from build123d import *

# Parameters (mm, degrees)
SKETCH_1_R              = 25
SKETCH_1_R_2            = 20
EXTRUDE_1_DEPTH         = 1
HOLE_WIZARD_3_9_3_9_1_D = 3.9
SKETCH_4_R              = 2
CUT_EXTRUDE_1_DEPTH     = 10


with BuildPart() as part:
    # 草图1 → 凸台-拉伸1 (new body)
    with BuildSketch(Plane.XY):
        with BuildLine():
            Line((-62.449979984, 62), (62.449979984, 62))
            ThreePointArc((62.449979984, 62), (0, -88), (-62.449979984, 62))
        make_face()
        Circle(SKETCH_1_R, mode=Mode.SUBTRACT)
        with Locations((54.772, 35)):
            Circle(SKETCH_1_R_2, mode=Mode.SUBTRACT)
        with Locations(Location((-54.772, 35, 0), (0, 0, 180))):
            Circle(SKETCH_1_R_2, mode=Mode.SUBTRACT)
        with Locations((35, -54.772255751)):
            Circle(SKETCH_1_R_2, mode=Mode.SUBTRACT)
        with Locations((-35, -54.772255751)):
            Circle(SKETCH_1_R_2, mode=Mode.SUBTRACT)
    extrude(amount=EXTRUDE_1_DEPTH)

    # Ø3.9 (3.9) 直径孔1 (through all)
    with Locations(Plane(origin=(0, 0, 0), x_dir=(-1, 0, 0), z_dir=(0, 0, -1))):
        with Locations((-77, 26), (-77, -27), (77, -27), (77, 26)):
            Hole(HOLE_WIZARD_3_9_3_9_1_D / 2)

    # 草图4 → 切除-拉伸1 (cut)
    with BuildSketch(Plane.XY.offset(1)):
        with Locations((-60, 0)):
            Circle(SKETCH_4_R)
        with Locations((0, 40)):
            Circle(SKETCH_4_R)
        with Locations((60, 0)):
            Circle(SKETCH_4_R)
        with Locations((0, -60)):
            Circle(SKETCH_4_R)
    extrude(amount=-CUT_EXTRUDE_1_DEPTH, mode=Mode.SUBTRACT)


solid = part.part
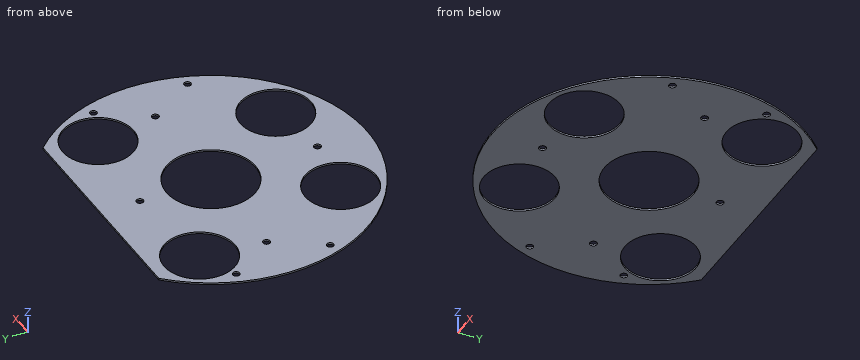
CAD build for the part. Positions are in the model's coordinates, mm. Round coordinates to 2 decimals unless told otherwise and drop trailing zeros. Order: outer loops, then holes, each group sorted by start corner. A loop starts at its lowest first (then second) coordinate and runs counter-clockwise, first axis right, second up. Notation, with made-up numbers: (14, 33) - (69, 33) arc R17 cw to (69, 57) - close; hole circle Ø5 at (-26, 15.5). An arc over 180 degrees is marked (long way). Return JSON: item names as keys, results as strings.
(1) Cut at C-C (y = -16.5). Give the cut face in (x, z), then the cut area to 3 significant figures.
Answer key:
{"outline": "(-86.44, 0) - (-18.78, 0) - (-18.78, 1) - (-86.44, 1) - close; (18.78, 0) - (86.44, 0) - (86.44, 1) - (18.78, 1) - close", "area": "135 mm^2"}
(2) Cut at D-D (z = 0.7). State how many separate pieces and enclosed holes the cut face has, then the cut area to 3 significant figures.
Answer key:
{"separate pieces": "1", "enclosed holes": "13", "area": "15,000 mm^2"}
(3) Pin check, flat tip, straight feed: pin 1 Ø3 at (x, y) = (0, -60) entering from -Z. Stop position of the tip, or through.
Answer key:
{"pin 1": "passes through"}
(4) Wall check: probe 1 along Y at (x, z) = (0, 0.2); probe 2 along X at (y, z) = (33.5, 0.4); probe 3 along X at (y, z) = (-68.5, 0.25). Give the ranges that are in metal, low to high. Write a range as from..to.
Answer key:
{"probe 1": "y = -88..-62, -58..-25, 25..38, 42..62", "probe 2": "x = -81.37..-74.72, -34.83..34.83, 74.72..81.37", "probe 3": "x = -55.24..-49.54, -20.46..20.46, 49.54..55.24"}
(5) Cut at B-B (x = 41). Give the cut face in (y, z).
Answer key:
{"outline": "(-77.87, 0) - (-73.85, 0) - (-73.85, 1) - (-77.87, 1) - close; (-35.69, 0) - (20.5, 0) - (20.5, 1) - (-35.69, 1) - close; (49.5, 0) - (62, 0) - (62, 1) - (49.5, 1) - close"}
(6) Cut at A-A (y = -60). Give the cut face in (x, z).
Answer key:
{"outline": "(-64.37, 0) - (-54.3, 0) - (-54.3, 1) - (-64.37, 1) - close; (-15.7, 0) - (-2, 0) - (-2, 1) - (-15.7, 1) - close; (2, 0) - (15.7, 0) - (15.7, 1) - (2, 1) - close; (54.3, 0) - (64.37, 0) - (64.37, 1) - (54.3, 1) - close"}
